The listing builds one solid part. Answer for the finished solid, in the listing's coordinates (mm). A direction names the side the tool comes from. Give positions to 0.01 mm unless a question says otherwise; leave off trailing zeros. Write each loop counter-clockwise with the first axis right and the second up, starting at its lowest first coordinate (ties: lowest second). Pieces come first, ordered by that corner, then holes. Notation, with made-up numbers: M 37,-14.5 L 73,-14.5 A19 ccw 73,2.5 Z; hole C -27,-10 d3. An arc over 180 degrees is marked long. Answer as a JSON object with one key per item and string values.
```python
from build123d import *

# Parameters (mm, degrees)
SKETCH_R    = 11.25
PAD_DEPTH   = 3
SKETCH001_R = 1.7
HOLE_DEPTH  = 25


with BuildPart() as part:
    # Sketch → Pad (new body)
    with BuildSketch(Plane.XY):
        Polygon((20.5, 21), (-20.5, 21), (-25, 16.5), (-25, -74.5), (-20.5, -79), (20.5, -79), (25, -74.5), (25, 16.5), align=None)
        Circle(SKETCH_R, mode=Mode.SUBTRACT)
        with BuildLine():
            ThreePointArc((-12.85, -39), (-15, -36.85), (-17.15, -39))
            Line((-17.15, -39), (-17.15, -68.5))
            ThreePointArc((-17.15, -68.5), (-15, -70.65), (-12.85, -68.5))
            Line((-12.85, -68.5), (-12.85, -39))
        make_face(mode=Mode.SUBTRACT)
        with BuildLine():
            ThreePointArc((17.15, -39), (15, -36.85), (12.85, -39))
            Line((12.85, -39), (12.85, -68.5))
            ThreePointArc((12.85, -68.5), (15, -70.65), (17.15, -68.5))
            Line((17.15, -68.5), (17.15, -39))
        make_face(mode=Mode.SUBTRACT)
    extrude(amount=PAD_DEPTH)

    # Sketch001 → Hole (cut)
    with BuildSketch(Plane.XY):
        with Locations((-15.5, 15.5)):
            Circle(SKETCH001_R)
        with Locations((15.5, 15.5)):
            Circle(SKETCH001_R)
        with Locations((15.5, -15.5)):
            Circle(SKETCH001_R)
        with Locations((-15.5, -15.5)):
            Circle(SKETCH001_R)
    extrude(amount=HOLE_DEPTH, mode=Mode.SUBTRACT)


solid = part.part
```
1. For faces 4 (the cylindrical face through (14.95, -70.65, 1.48)), 5 (the flat face through (-25, -28, 1)), determine the directions among +Z, -Z, +X, -X, +Y, -Y from which every point of the face is accessible in a straight line to the end or side of a thin tool.
Verdict:
{"face 4": "+Z, -Z", "face 5": "+Z, -Z, -X, +Y, -Y"}
2. Consider line 1 along X through (y, z) = (-15.5, 1.55); line 2 along Y through (x, z) = (-15.5, 0.95); line 3 along Y through (x, z) = (-4, 2.05). Determine where each line is inside the solid, lowest interval first.
Verdict:
{"line 1": "x = -25 to -17.2, -13.8 to 13.8, 17.2 to 25", "line 2": "y = -79 to -70.59, -36.91 to -17.2, -13.8 to 13.8, 17.2 to 21", "line 3": "y = -79 to -10.51, 10.51 to 21"}
3. The mould has two halves that part along X. Classify faces 1 (the cylindrical face through (17.07, 14.85, 1.48)), 2 (the flat face through (0, -28, 3)), 3 (the flat face through (22.7, -76.8, 1.5)): released by +X, released by -X, zero draft, split by the parting line, or undercut.
Verdict:
{"face 1": "undercut", "face 2": "zero draft", "face 3": "released by +X"}
4. A cutting plane is placed at B-B, the plane y = 0. Give the vertices of the cut face in (x, z), plus the area to 3 significant figures.
Verdict:
{"outline": "M -25,0 L -11.25,0 L -11.25,3 L -25,3 Z; M 11.25,0 L 25,0 L 25,3 L 11.25,3 Z", "area": "82.5 mm2"}
5. A cutting plane is placed at C-C, the plane y = -43.5. Give the vertices of the cut face in (x, z).
Verdict:
{"outline": "M -25,0 L -17.15,0 L -17.15,3 L -25,3 Z; M -12.85,0 L 12.85,0 L 12.85,3 L -12.85,3 Z; M 17.15,0 L 25,0 L 25,3 L 17.15,3 Z"}
6. A cutting plane is placed at A-A, the plane x = 0. Give the vertices of the cut face in (y, z), plus the area to 4 significant figures.
Verdict:
{"outline": "M -79,0 L -11.25,0 L -11.25,3 L -79,3 Z; M 11.25,0 L 21,0 L 21,3 L 11.25,3 Z", "area": "232.5 mm2"}
7. A cutting plane is placed at D-D, the plane z = 0.9. Give the vertices of the cut face in (x, y), plus the area to 3 significant figures.
Verdict:
{"outline": "M -25,-74.5 L -20.5,-79 L 20.5,-79 L 25,-74.5 L 25,16.5 L 20.5,21 L -20.5,21 L -25,16.5 Z; hole C -15.5,-15.5 d3.4; hole C -15.5,15.5 d3.4; hole M -17.15,-68.5 A2.15 ccw -12.85,-68.5 L -12.85,-39 A2.15 ccw -17.15,-39 Z; hole C 0,0 d22.5; hole M 12.85,-68.5 A2.15 ccw 17.15,-68.5 L 17.15,-39 A2.15 ccw 12.85,-39 Z; hole C 15.5,-15.5 d3.4; hole C 15.5,15.5 d3.4", "area": "4,240 mm2"}
